Geometry check sheet. Reference: the model listing, model coordinates, mm. A direction names the side the tool comes from. Give positions to 0.01 mm unless a question says otherwise; leave off trailing zeros. Order: outer loops, then holes, each group sorted by start corner. A loop starts at its lowest first (then second) coordinate and runs counter-clockwise, first axis right, second up. Notation, with made-up numbers: M 13,17.25 L 67,17.25 A16 ccw 67,29.25 Z; hole C -7,-15 d2. An arc over 180 degrees is marked long. Put each result on its own line as item: value. Start each with the question number.
Q1. Go/stop test with flat-tipped pins: pin 1 (1.6 mm diameter, centred on x = -7.5, z = 2, fed in from +Y); pin 2 (1 mm diameter, centred on y = 14.5, z = 1.5, fed in from -X); pin 3 (2 mm diameter, centred on x = -54.5, y = 22.5, fed in from -Z); pin 4 (1.6 mm diameter, centred on x = 1.5, z = 1.5, fed in from -Y). Record where each tip stops, or that it passes through.
Q2. Access from +Z, -Z, +X, -X, +Y, -Y to the whole of each face (thin tool, end or side, straight path). Record for faces 4 (the cylindrical face through (48.932, -50.464, 1.565)), 5 (the cylindrical face through (54.023, 3.67, 1.565)).
Q3. Material ranges on L1, parallel to X at y = -40, z = 0.85; L2, parallel to Y at x = -140.5, z = 0.3; L3, parallel to X at y = 60, z = 1.65, recorded low to high.
Q4. Section check D-D on y = -50.5. Record the cut outline in (x, z) (1 decimal).
Q5. Mould release check, pull along X, two halves, no side actions. Record for faces 1 (the flat face through (-18, -6, 3.175)), 2 (the cylindrical face through (49.83, 50.8, 1.57)), 3 (the cylindrical face through (-48.934, 50.464, 1.565)): +X half, -X half, draft (parallel to the pull), parting line (faces both ways), or undercut.
Q6. Section check A-A on y = 0. Record the cut outline in (x, z) (3 decimals), then the cut area to 3 significant figures.
Q7. Section check C-C on x = -178.5. Record the cut outline in (y, z) (3 decimals).
Q8. Section check B-B on z = 1.5. Record the cut outline in (x, y) (3 decimals).
```python
from build123d import *

# Parameters (mm, degrees)
SKETCH1_R           = 83.4771
SKETCH1_R_2         = 3.175
BOSS_EXTRUDE1_DEPTH = 3.175
SKETCH2_W           = 25.4
SKETCH2_H           = 25.4
CUT_EXTRUDE1_DEPTH  = 4.175
SKETCH3_W           = 76.2
SKETCH3_H           = 3.175
CUT_EXTRUDE2_DEPTH  = 4.175


with BuildPart() as part:
    # Sketch1 → Boss-Extrude1 (new body)
    with BuildSketch(Plane.XY):
        with BuildLine():
            Line((-15.854735322, -44.594342032), (15.852600775, -44.594342032))
            ThreePointArc((15.852600775, -44.594342032), (49.382027762, -50.630069264), (78.701832464, -67.979464917))
            ThreePointArc((78.701832464, -67.979464917), (227.246053, 0), (78.701832464, 67.979464917))
            ThreePointArc((78.701832464, 67.979464917), (49.382027762, 50.630069264), (15.852600775, 44.594342032))
            Line((15.852600775, 44.594342032), (-15.854735322, 44.594342032))
            ThreePointArc((-15.854735322, 44.594342032), (-49.384162309, 50.630069264), (-78.703967011, 67.979464917))
            ThreePointArc((-78.703967011, 67.979464917), (-227.248187547, 0), (-78.703967011, -67.979464917))
            ThreePointArc((-78.703967011, -67.979464917), (-49.384162309, -50.630069264), (-15.854735322, -44.594342032))
        make_face()
        with Locations((137.418953, 0)):
            Circle(SKETCH1_R, mode=Mode.SUBTRACT)
        with Locations((-137.421087547, 0)):
            Circle(SKETCH1_R, mode=Mode.SUBTRACT)
        with Locations((0, 28.575000036)):
            Circle(SKETCH1_R_2, mode=Mode.SUBTRACT)
    extrude(amount=BOSS_EXTRUDE1_DEPTH)

    # Sketch2 → Cut-Extrude1 (cut, through all)
    with BuildSketch(Plane.XY.offset(3.175)):
        with Locations((0, 28.575000036)):
            Rectangle(SKETCH2_W, SKETCH2_H)
    extrude(amount=-CUT_EXTRUDE1_DEPTH, mode=Mode.SUBTRACT)

    # Sketch3 → Cut-Extrude2 (cut, through all)
    with BuildSketch(Plane.XY.offset(3.175)):
        with Locations((0, 14.287500036)):
            Rectangle(SKETCH3_W, SKETCH3_H)
    extrude(amount=-CUT_EXTRUDE2_DEPTH, mode=Mode.SUBTRACT)


solid = part.part
```
Results found:
1. pin 1: stops at y = 44.59
1. pin 2: stops at x = -226.15
1. pin 3: stops at z = 0
1. pin 4: stops at y = -44.59
2. face 4: +Z, -Z, -Y
2. face 5: +Z, -Z
3. L1: x = -217.85 to -210.69, -64.15 to 64.15, 210.69 to 217.85
3. L2: y = -89.77 to -83.42, 83.42 to 89.77
3. L3: x = -204.27 to -195.46, -79.38 to -68.06, 68.06 to 79.38, 195.46 to 204.27
4. outline: M -211.7,0 L -203.9,0 L -203.9,3.2 L -211.7,3.2 Z; M -71,0 L -49,0 L -49,3.2 L -71,3.2 Z; M 49,0 L 70.9,0 L 70.9,3.2 L 49,3.2 Z; M 203.9,0 L 211.7,0 L 211.7,3.2 L 203.9,3.2 Z
5. face 1: draft
5. face 2: undercut
5. face 3: undercut
6. outline: M -227.248,0 L -220.898,0 L -220.898,3.175 L -227.248,3.175 Z; M -53.944,0 L 53.942,0 L 53.942,3.175 L -53.944,3.175 Z; M 220.896,0 L 227.246,0 L 227.246,3.175 L 220.896,3.175 Z
6. area: 383 mm^2
7. outline: M -79.884,0 L -72.67,0 L -72.67,3.175 L -79.884,3.175 Z; M 72.67,0 L 79.884,0 L 79.884,3.175 L 72.67,3.175 Z
8. outline: M -78.704,-67.979 A96.149 cw -15.855,-44.594 L 15.853,-44.594 A96.149 cw 78.702,-67.979 A89.827 ccw long 78.702,67.979 A96.149 cw 15.853,44.594 L -15.855,44.594 A96.149 cw -78.704,67.979 A89.827 ccw long Z; hole C -137.421,0 d166.954; hole M -38.1,12.7 L 38.1,12.7 L 38.1,15.875 L 12.7,15.875 L 12.7,41.275 L -12.7,41.275 L -12.7,15.875 L -38.1,15.875 Z; hole C 137.419,0 d166.954
